Check sheet for the modelled part. Datum: model origin and axes. Units: mm. A direction names the side the tool comes from. Give positions to 0.01 mm unless a question says otherwise; leave off trailing zeros. Loops run counter-clockwise (first coordinate to the right, second up) from the corner with the lowest first, then second, coordinate; pieces in that order, holes last.
```python
from build123d import *

# Parameters (mm, degrees)
BOSS_EXTRUDE1_DEPTH   = 3
BOSS_EXTRUDE2_DEPTH   = 3.7
BOSS_EXTRUDE3_DEPTH   = 3
SKETCH4_R             = 2.88
BOSS_EXTRUDE4_DEPTH   = 12
F_2_5MM_DOWEL_HOLE1_D = 2.5
SKETCH8_R             = 1.35
CUT_EXTRUDE1_DEPTH    = 38.455173265
FILLET1_R             = 1
FILLET2_R             = 1
FILLET3_R             = 0.5


with BuildPart() as part:
    # Sketch1 → Boss-Extrude1 (new body)
    with BuildSketch(Plane(origin=(0, 0, 0), x_dir=(1, 0, 0), z_dir=(0, 1, 0))):
        with BuildLine():
            Line((0, 13), (16, 13))
            Line((16, 13), (16, 7))
            Line((16, 7), (0, 7))
            ThreePointArc((0, 7), (-7, 0), (0, -7))
            Line((0, -7), (16, -7))
            Line((16, -7), (16, -13))
            Line((16, -13), (0, -13))
            ThreePointArc((0, -13), (-13, 0), (0, 13))
        make_face()
    extrude(amount=BOSS_EXTRUDE1_DEPTH)

    # Sketch2 → Boss-Extrude2 (add)
    with BuildSketch(Plane(origin=(0, 3, 0), x_dir=(1, 0, 0), z_dir=(0, 1, 0))):
        with BuildLine():
            Line((0, 13), (16, 13))
            Line((16, 13), (16, 10))
            Line((16, 10), (0, 10))
            ThreePointArc((0, 10), (-10, 0), (0, -10))
            Line((0, -10), (16, -10))
            Line((16, -10), (16, -13))
            Line((16, -13), (0, -13))
            ThreePointArc((0, -13), (-13, 0), (0, 13))
        make_face()
    extrude(amount=BOSS_EXTRUDE2_DEPTH)

    # Sketch3 → Boss-Extrude3 (add)
    with BuildSketch(Plane(origin=(0, 6.7, 0), x_dir=(1, 0, 0), z_dir=(0, 1, 0))):
        with BuildLine():
            Line((16, 13), (0, 13))
            ThreePointArc((0, 13), (-13, 0), (0, -13))
            Line((0, -13), (16, -13))
            Line((16, -13), (16, -7))
            Line((16, -7), (16, 7))
            Line((16, 7), (16, 13))
        make_face()
    extrude(amount=BOSS_EXTRUDE3_DEPTH)

    # Sketch4 → Boss-Extrude4 (add)
    with BuildSketch(Plane(origin=(0, 9.7, 0), x_dir=(1, 0, 0), z_dir=(0, 1, 0))):
        with Locations(Location((0, 0, 0), (0, 0, 270))):
            Circle(SKETCH4_R)
    extrude(amount=BOSS_EXTRUDE4_DEPTH)

    # Ø2.5mm Dowel Hole1 (through all)
    with Locations(Plane(origin=(-0.002429038, 18.104937254, 2.879998976), x_dir=(0.999999644325, 0, 0.000843415861), z_dir=(-0.000843415861, 0, 0.999999644325))):
        with Locations((0, 0)):
            Hole(F_2_5MM_DOWEL_HOLE1_D / 2)

    # Sketch8 → Cut-Extrude1 (cut, through all)
    with BuildSketch(Plane.XY.offset(13)):
        with Locations((12.5, 4.85)):
            Circle(SKETCH8_R)
    extrude(amount=-CUT_EXTRUDE1_DEPTH, mode=Mode.SUBTRACT)

    # Fillet1
    fillet1_edges = [part.edges().sort_by_distance(p)[0] for p in [
        (8, 0, -13),
        (8, 0, -7),
        (-7, 0, 0),
        (16, 4.85, 13),
        (-13, 9.7, 0),
        (8, 9.7, 13),
        (8, 9.7, -13),
        (8, 0, 7),
        (8, 0, 13),
        (-13, 0, 0),
    ]]
    fillet(fillet1_edges, radius=FILLET1_R)

    # Fillet2
    fillet2_edges = [part.edges().sort_by_distance(p)[0] for p in [
        (0, 9.7, -2.88),
    ]]
    fillet(fillet2_edges, radius=FILLET2_R)

    # Fillet3
    fillet3_edges = [part.edges().sort_by_distance(p)[0] for p in [
        (0, 21.7, -2.88),
    ]]
    fillet(fillet3_edges, radius=FILLET3_R)


solid = part.part
```
(1) Access from +Z, -Z, +X, -X, +Y, -Y to the whole of each face (thin tool, end or side, straight path). Record for faces 1 (the face through (8, 2, 7)), 2 (the face through (8, 5, -10)), 3 (the face through (8.112, 9.415, 12.699)).
(2) Release check for a two-part mould opening along Y. For faces 4 (the face through (3, 6.7, 0)), 5 (the face through (5, 9.7, 0)), 6 (the face through (15.715, 4.782, 12.699)), 7 (the face through (7.888, 0.301, 12.715)) record: pulls with the +Y half, pulls with the -Y half, needs draft (parallel to the pull), parting line crosses it, or undercut.
(3) Section check B-B on y = 4.25. Record the boundary of the cut face in (x, z).
(4) Section check C-C on y = 8.25. Record the boundary of the cut face in (x, z).
(5) Section check A-A on x = 12.5. Record the boundary of the cut face in (y, z), plus the area to 3 significant figures.
(6) Section check D-D on y = 11.75. Record the boundary of the cut face in (x, z).
(7) Gauge pin test, flat ends, axial feed: pin 1 Ø12 at (x, z) = (-8.5, -5) entering from +Y; pin 2 Ø2 at (x, y) = (12.5, 4.85) entering from +Z; pin 3 Ø1 at (x, y) = (0, 17) entering from +Z. Record the tip position at first contact, or that the pin passes through.
(8) Material ranges on line 1 (Y direction, x = 12.5, z = -11.15); line 2 (Z direction, x = 5.5, y = 1.5); line 3 (Y direction, x = 7.5, z = 5.5), recorded low to high.
Computed values:
1. face 1: +X, -Y
1. face 2: +X
1. face 3: +Z, +X, -X, +Y
2. face 4: undercut
2. face 5: pulls with the +Y half
2. face 6: needs draft
2. face 7: pulls with the -Y half
3. outline: (0, -13) - (11.29, -13) - (11.29, -10) - (0, -10) arc R10 cw to (0, 10) - (11.29, 10) - (11.29, 13) - (0, 13) arc R13 ccw to start; (13.71, -13) - (16, -13) - (16, -10) - (13.71, -10) - close; (13.71, 10) - (16, 10) - (16, 12) arc R1 ccw to (15, 13) - (13.71, 13) - close
4. outline: (0, -13) - (16, -13) - (16, 12) arc R1 ccw to (15, 13) - (0, 13) arc R13 ccw to start
5. outline: (0, -12) arc R1 ccw to (1, -13) - (3.5, -13) - (3.5, -10) - (3, -10) - (3, -7) - (1, -7) arc R1 ccw to (0, -8) - close; (0, 8) arc R1 ccw to (1, 7) - (3, 7) - (3, 10) - (3.5, 10) - (3.5, 13) - (1, 13) arc R1 ccw to (0, 12) - close; (6.2, -13) - (8.7, -13) arc R1 ccw to (9.7, -12) - (9.7, 12) arc R1 ccw to (8.7, 13) - (6.2, 13) - (6.2, 10) - (6.7, 10) - (6.7, -10) - (6.2, -10) - close
5. area: 119 mm2
6. outline: circle Ø5.76 at (0, 0)
7. pin 1: stops at y = 9.7
7. pin 2: passes through
7. pin 3: stops at z = 2.88
8. line 1: y = 0 to 3.5, 6.2 to 9.7
8. line 2: z = -13 to -7, 7 to 13
8. line 3: y = 6.7 to 9.7
